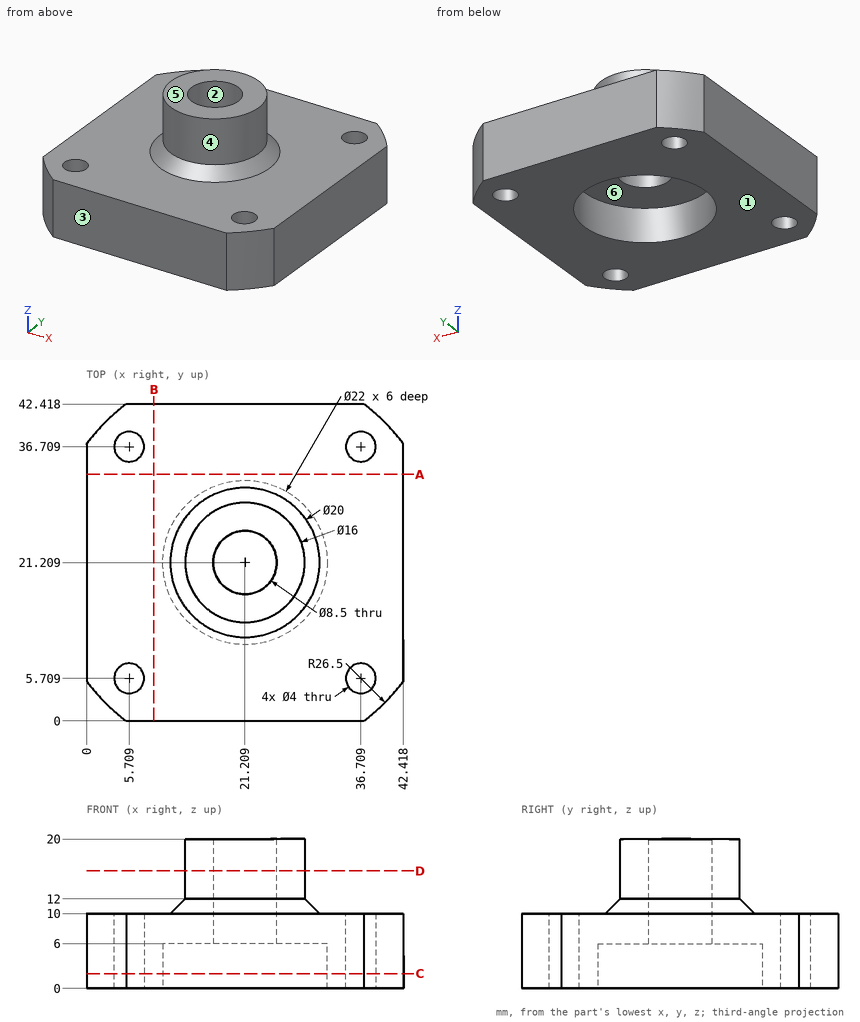
Geometry: see drawing. Coordinates: mm, zero at the bounding-box minimum. A direction names the side the tool comes from. Round coordinates to 2 decimals unless told otherwise and drop trailing zeros. Order: outer loops, then holes, each group sorted by start corner. A loop starts at its lowest first (then second) coordinate and runs counter-clockwise, first axis right, second up. Notation, with made-up numbers: (-23, -15) -> (18, -15) arc R26 cw to (18, 18) -> close; hole circle Ø4 at (30.25, 87). An arc over 180 degrees is marked (long way). Answer as CSV lines item,"result".
Item 1: Section A-A, the plane y = 33. Return loops of the section in (x, z).
A:
outline,"(0, 0) -> (42.42, 0) -> (42.42, 10) -> (0, 10) -> close"
Item 2: Line query: L1, parallel to Z at x = 11, y = 4.5; L2, parallel to Y at x = 17.5, z = 7; L3, parallel to Y at x = 17.5, z = 14.5. Output: solid intervals per line, ascending.
A:
L1,"0 to 10"
L2,"0 to 19.13, 23.28 to 42.42"
L3,"14.12 to 19.13, 23.28 to 28.3"
Item 3: Pin query (flat end, axial travel): pin 1 Ø17.5 at (x, y) = (20, 22) entering from -Z; pin 2 Ø3 at (y, z) = (25, 14) entering from -X; pin 3 Ø6.5 at (x, y) = (36.709, 5.709) entering from +Z. Return the tip coordinate at first contact, or that it passes through.
A:
pin 1,"z = 6"
pin 2,"x = 13.54"
pin 3,"z = 10"
Item 4: Section D-D, the plane z = 15.75. Return loops of the section in (x, y), plus the area to 3 significant figures.
A:
outline,"circle Ø16 at (21.21, 21.21); hole circle Ø8.5 at (21.21, 21.21)"
area,"144 mm²"
Item 5: Section C-C, the plane z = 2. Count the separate pieces of the cut face and the enclosed holes in it, plus the area to 3 significant figures.
A:
separate pieces,"1"
enclosed holes,"5"
area,"1,320 mm²"
Item 6: Reachability of the marked faces 4, 5 and 6 from +Z, -Z, +X, -X, +Y, -Y: full face, straight path, thin tool, end or side. Return the list, or none.
A:
face 4,"+Z"
face 5,"+Z, +X, -X, +Y, -Y"
face 6,"-Z"
Item 7: Pull-direction query (Y, two-part tool) for the marked faces 1, 2 and 3; classes: pulls with the +Y half, pulls with the -Y half, needs draft (parallel to the pull), parting line crosses it, or undercut.
A:
face 1,"needs draft"
face 2,"undercut"
face 3,"pulls with the -Y half"
